```python
from build123d import *

# Parameters (mm, degrees)
SKETCH_1_W          = 50
SKETCH_1_H          = 15
EXTRUDE_1_DEPTH     = 2
FILLET_1_R          = 5
FILLET_2_R          = 7.5
SKETCH_3_R          = 1.5
SKETCH_3_R_2        = 2
CUT_EXTRUDE_1_DEPTH = 2
SKETCH_4_R          = 1.5
CUT_EXTRUDE_2_DEPTH = 10


with BuildPart() as part:
    # 草图1 → 凸台-拉伸1 (new body)
    with BuildSketch(Plane.XY):
        Rectangle(SKETCH_1_W, SKETCH_1_H)
    extrude(amount=EXTRUDE_1_DEPTH)

    # 圆角1
    fillet_1_edges = [part.edges().sort_by_distance(p)[0] for p in [
        (-25, -7.5, 1),
        (-25, 7.5, 1),
    ]]
    fillet(fillet_1_edges, radius=FILLET_1_R)

    # 圆角2
    fillet_2_edges = [part.edges().sort_by_distance(p)[0] for p in [
        (25, -7.5, 1),
        (25, 7.5, 1),
    ]]
    fillet(fillet_2_edges, radius=FILLET_2_R - 0.0001)  # a hair under: the kernel refuses the full size

    # 草图3 → 切除-拉伸1 (cut)
    with BuildSketch(Plane.XY.offset(2)):
        with Locations((-20, 2.5)):
            Circle(SKETCH_3_R)
        with Locations((-12.482459034, -0.236161147)):
            Circle(SKETCH_3_R)
        with Locations((17.5, 0)):
            Circle(SKETCH_3_R_2)
    extrude(amount=-CUT_EXTRUDE_1_DEPTH, mode=Mode.SUBTRACT)

    # 草图4 → 切除-拉伸2 (cut)
    with BuildSketch(Plane.XY.offset(2)):
        with Locations((3.310591225, -1.5)):
            Circle(SKETCH_4_R)
    extrude(amount=-CUT_EXTRUDE_2_DEPTH, mode=Mode.SUBTRACT)


solid = part.part
```
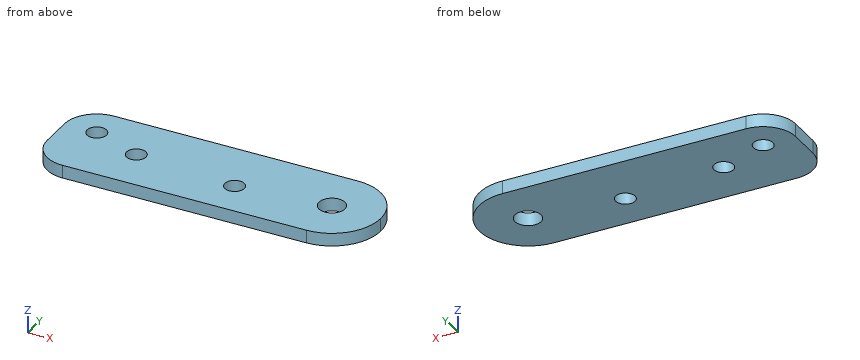
Geometry check sheet. Reference: the model listing, model coordinates, mm. Round coordinates to 2 decimals unless told otherwise and drop trailing zeros. Loops run counter-clockwise (first coordinate to the right, second up) from the corner with the lowest first, then second, coordinate; pieces in that order, holes last. Notation, with made-up numbers: (9.25, 81) - (25.25, 81) arc R7 ccw to (25.25, 88) - close; hole circle Ø7 at (-38, 77). An arc over 180 degrees is marked (long way). Write each question's results on one line, items separated by ' | '. Start each with the question number.
Q1. Cross-section at C-C on y = -5.75. Enter the section's corners in (x, z).
Q2. Cross-section at A-A on z = 0.9. State how many separate pieces and enclosed holes the cut face has, and give its area (3 significant figures).
Q3. Thickness scan on line 1 (Y direction, x = 17.5, z = 1); line 2 (Y direction, x = -20, z = 1.1); line 3 (X direction, y = -0.75, z = 1.75). Record the ranges inside material, lowest first. Write a range as [from, to].
Q4. Cross-section at B-B on x = -19. Enter the section's corners in (y, z).
Q5. Cross-section at D-D on y = 4.75. Enter the section's corners in (x, z), and give its area (3 significant figures).
Answers below:
1) outline: (-23.8, 0) - (22.32, 0) - (22.32, 2) - (-23.8, 2) - close
2) separate pieces: 1 | enclosed holes: 4 | area: 681 mm²
3) line 1: y = [-7.5, -2], [2, 7.5] | line 2: y = [-7.5, 1], [4, 7.5] | line 3: x = [-25, -13.89], [-11.07, 2.01], [4.61, 15.65], [19.35, 24.96]
4) outline: (-7.5, 0) - (1.38, 0) - (1.38, 2) - (-7.5, 2) - close; (3.62, 0) - (7.5, 0) - (7.5, 2) - (3.62, 2) - close
5) outline: (-24.47, 0) - (23.3, 0) - (23.3, 2) - (-24.47, 2) - close | area: 95.5 mm²
